Can you work these out from the model? Positions are in its coordinate system, mm. Give positions to 0.01 mm unless a question says otherwise; leave off trailing zeros. Write each question's results on one line, items separated by ' | '.
from build123d import *

# Parameters (mm, degrees)
GENERALSHAPE_DEPTH           = 0.8
ADDTOLERANCE_DEPTH           = 71.715203457
ADDTOLERANCE_DEPTH_BACK      = 71.715203457
BACKPLANE_DEPTH              = 71.573791169
BACKPLANE_DEPTH_BACK         = 71.573791169
RF_W                         = 3.18
RF_H                         = 4.2
CUT_EXTRUDE1_DEPTH           = 71.587392642
FILLET1_R                    = 1.27
F_0_32_0_32_DIAMETER_HOLE1_D = 0.32


with BuildPart() as part:
    # Sketch2 → GeneralShape (new, symmetric)
    with BuildSketch(Plane(origin=(0, 0, 0), x_dir=(1, 0, 0), z_dir=(0, 1, 0))):
        Polygon((47.4, 46.4), (37, 46.4), (37, 50), (-37, 50), (-37, 46.4), (-47.4, 46.4), (-47.4, 41.5), (-50, 41.5), (-50, -41.5), (-47.4, -41.5), (-41.5, -47.4), (41.5, -47.4), (47.4, -41.5), (50, -41.5), (50, 41.5), (47.4, 41.5), align=None)
    extrude(amount=GENERALSHAPE_DEPTH, both=True)

    # Sketch3 → AddTolerance (cut, two sides: drawn at the far end of the back side and taken through both)
    with BuildSketch(Plane(origin=(0, 0, 0), x_dir=(1, 0, 0), z_dir=(0, 1, 0)).offset(-ADDTOLERANCE_DEPTH_BACK)):
        Polygon((37, 50), (-37, 50), (-37, 46.4), (-47.4, 46.4), (-47.4, 41.5), (-50, 41.5), (-50, -41.5), (-47.4, -41.5), (-47.5, -41.4), (-49.9, -41.4), (-49.9, 41.4), (-47.3, 41.4), (-47.3, 46.3), (-36.9, 46.3), (-36.9, 49.9), (36.9, 49.9), (36.9, 46.3), (47.3, 46.3), (47.3, 41.4), (49.9, 41.4), (49.9, -41.4), (47.5, -41.4), (47.4, -41.5), (50, -41.5), (50, 41.5), (47.4, 41.5), (47.4, 46.4), (37, 46.4), align=None)
    extrude(amount=ADDTOLERANCE_DEPTH + ADDTOLERANCE_DEPTH_BACK, mode=Mode.SUBTRACT)

    # Sketch4 → Backplane (cut, two sides: drawn at the far end of the back side and taken through both)
    with BuildSketch(Plane(origin=(0, 0, 0), x_dir=(1, 0, 0), z_dir=(0, 1, 0)).offset(-BACKPLANE_DEPTH_BACK)):
        with BuildLine():
            Line((41.5, -47.4), (44.1, -44.8))
            Line((44.1, -44.8), (41.232050808, -44.8))
            ThreePointArc((41.232050808, -44.8), (39.5, -43.8), (37.767949192, -44.8))
            Line((37.767949192, -44.8), (18.232050808, -44.8))
            ThreePointArc((18.232050808, -44.8), (16.5, -43.8), (14.767949192, -44.8))
            Line((14.767949192, -44.8), (-14.767949192, -44.8))
            ThreePointArc((-14.767949192, -44.8), (-16.5, -43.8), (-18.232050808, -44.8))
            Line((-18.232050808, -44.8), (-37.767949192, -44.8))
            ThreePointArc((-37.767949192, -44.8), (-39.5, -43.8), (-41.232050808, -44.8))
            Line((-41.232050808, -44.8), (-44.1, -44.8))
            Line((-44.1, -44.8), (-41.5, -47.4))
            Line((-41.5, -47.4), (41.5, -47.4))
        make_face()
    extrude(amount=BACKPLANE_DEPTH + BACKPLANE_DEPTH_BACK, mode=Mode.SUBTRACT)

    # RF → Cut-Extrude1 (cut, through all)
    with BuildSketch(Plane(origin=(0, 0.8, 0), x_dir=(1, 0, 0), z_dir=(0, 1, 0))):
        with Locations((-22, -38.7)):
            Rectangle(RF_W, RF_H)
        with Locations((-28, -38.7)):
            Rectangle(RF_W, RF_H)
        with Locations((-34, -38.7)):
            Rectangle(RF_W, RF_H)
        with BuildLine():
            Line((-18.232050808, -40.8), (-20.41, -40.8))
            Line((-20.41, -40.8), (-23.59, -40.8))
            Line((-23.59, -40.8), (-26.41, -40.8))
            Line((-26.41, -40.8), (-29.59, -40.8))
            Line((-29.59, -40.8), (-32.41, -40.8))
            Line((-32.41, -40.8), (-35.59, -40.8))
            Line((-35.59, -40.8), (-37.767949192, -40.8))
            Line((-37.767949192, -40.8), (-37.767949192, -43.8))
            Line((-37.767949192, -43.8), (-39.5, -43.8))
            ThreePointArc((-39.5, -43.8), (-38.5, -44.067949192), (-37.767949192, -44.8))
            Line((-37.767949192, -44.8), (-18.232050808, -44.8))
            ThreePointArc((-18.232050808, -44.8), (-17.5, -44.067949192), (-16.5, -43.8))
            Line((-16.5, -43.8), (-18.232050808, -43.8))
            Line((-18.232050808, -43.8), (-18.232050808, -40.8))
        make_face()
    extrude(amount=-CUT_EXTRUDE1_DEPTH, mode=Mode.SUBTRACT)

    # Fillet1
    fillet1_edges = [part.edges().sort_by_distance(p)[0] for p in [
        (-23.59, 0, 36.6),
        (-20.41, 0, 36.6),
        (-18.232050808, 0, 40.8),
        (-37.767949192, 0, 40.8),
        (-35.59, 0, 36.6),
        (-32.41, 0, 36.6),
        (-29.59, 0, 36.6),
        (-26.41, 0, 36.6),
    ]]
    fillet(fillet1_edges, radius=FILLET1_R)

    # Ø0.32 (0.32) Diameter Hole1 (through all)
    with Locations(Plane(origin=(0, 0.8, 0), x_dir=(1, 0, 0), z_dir=(0, 1, 0))):
        with Locations((-20.41, -36.6), (-23.59, -36.6), (-26.41, -36.6), (-29.59, -36.6), (-32.41, -36.6), (-35.59, -36.6)):
            Hole(F_0_32_0_32_DIAMETER_HOLE1_D / 2)


solid = part.part
(1) We'd pull the mould along Z, two halves only. Please class faces 1 (the face through (-45.8, 0, 43.1)), 2 (the face through (-1, 0.8, -3)): +Z half, -Z half, draft (parallel to the pull), parting line (faces both ways), or undercut.
Data:
face 1: +Z half | face 2: draft
(2) I need wall thicknesses on L1, parallel to Z at x = -21.5, y = -0.45; L2, parallel to Z at x = -31.5, y = 0.6. Which ranges of each line are inside material? Lowest first, please. Write a range as from..to.
Data:
L1: z = -49.9..36.61 | L2: z = -49.9..40.8
(3) Imagine slicing it at A-A, the plane y = -0.2. Count the separate pieces of the cut face and the enclosed holes in it, plus the area to 3 significant figures.
Data:
separate pieces: 1 | enclosed holes: 6 | area: 9,180 mm2
(4) Will these pins go through, and if not, where does the flat tip stop? P1, Ø0.5, axis at x = 48.5, y = 0, coming from the +Z side; P2, Ø0.5, axis at x = 42.5, y = 0, coming from the -Z side.
Data:
P1: stops at z = 41.4 | P2: stops at z = -46.3
